Autodesk Inventor part; units mm, degrees
ref_plane "YZ Plane" through (0, 0, 0) normal (1, 0, 0) x (0, 1, 0)
ref_plane "XZ Plane" through (0, 0, 0) normal (0, 1, 0) x (-1, 0, 0)
ref_plane "XY Plane" through (0, 0, 0) normal (0, 0, 1) x (1, 0, 0)
sketch "Sketch1" plane through (0, 0, 0) normal (0, 1, 0) x (-1, 0, 0)
  circle A0 centre (0, -24) radius 19
  point P0 (0, 0)
  dimension "d1" = 38
  dimension "d3" = 24
extrude "Extrusion1" add sketch "Sketch1" along normal blind 1
sketch "Sketch3" plane through (0, 1, -24) normal (0, 1, 0) x (1, 0, 0)
  circle A0 centre (0, 0) radius 14
  circle A1 centre (0, 0) radius 19
  circle A2 centre (0, 0) radius 19
  point P0 (0, -24)
  dimension "d7" = 28
extrude "Extrusion3" add sketch "Sketch3" along normal blind 22 contours A0
sketch "Sketch5" plane through (0, 23, -24) normal (0, 1, 0) x (1, 0, 0)
  circle A0 centre (0, 0) radius 19
  point P0 (0, -24)
extrude "Extrusion5" add sketch "Sketch5" along normal blind 1
properties part number "flywheels"
Verification items for the finished model (mm, model axes). A direction names the side the tool comes from. Coordinates: 2 decimals unless noted, no trailing zeros. Loops run counter-clockwise (first coordinate to the right, second up) from the corner with the lowest first, then second, coordinate; pieces in that order, holes last. Notation, with made-up numbers: (2.5, 55) -> (13.5, 55) arc R25 ccw to (13.5, 73) -> close; hole circle Ø2 at (-30, 68.5). An arc over 180 degrees is marked (long way). Answer in a Markdown table with one row per item. Add a question column.
1. Access from +Z, -Z, +X, -X, +Y, -Y to the whole of each face (thin tool, end or side, straight path). Record for faces 1 (the face through (9, 1, -35)), 2 (the face through (0, 24, -24)).
2. Section check D-D, the plane z = -9. Enter the section's corners in (x, y).
3. Section check B-B, the plane x = 0. Enter the section's corners in (y, z).
4. Draft check along Y on faces 3 (the face through (-3.03, 11.85, -37.67)), 4 (the face through (0, 0, -24)), 5 (the face through (-10.214, 0.493, -40.021)). Enter one of: +Y half, -Y half, draft (parallel to the pull), parting line (faces both ways), or undercut.
5. Section check C-C, the plane y = 16.5. Enter the section's corners in (x, z).
6. Section check A-A, the plane z = -24. Enter the section's corners in (x, y), then the cut area to 3 significant figures.
7. Material ranges on probe 1 along Y at (x, z) = (9, -11); probe 2 along X at (y, z) = (12, -11); probe 3 along X at (y, z) = (19.5, -29), recorded low to high. Write a range as [from, to].
8. Depth check by flat-ended pin: P1, Ø1, axis at y = 8.5, z = -33.5, coming from the +X side; P2, Ø4, axis at x = 10.5, y = 5, coming from the -Z side; P3, Ø3, axis at y = 7.5, z = -21.5, coming from the -X side. Enter the tip coordinate at first touch or a pass-through.
Derived:
| question | item | result |
|---|---|---|
| 1 | face 1 | none |
| 1 | face 2 | +Z, -Z, +X, -X, +Y |
| 2 | outline | (-11.66, 0) -> (11.66, 0) -> (11.66, 1) -> (-11.66, 1) -> close; (-11.66, 23) -> (11.66, 23) -> (11.66, 24) -> (-11.66, 24) -> close |
| 3 | outline | (0, -43) -> (1, -43) -> (1, -38) -> (23, -38) -> (23, -43) -> (24, -43) -> (24, -5) -> (23, -5) -> (23, -10) -> (1, -10) -> (1, -5) -> (0, -5) -> close |
| 4 | face 3 | undercut |
| 4 | face 4 | -Y half |
| 4 | face 5 | draft |
| 5 | outline | circle Ø28 at (0, -24) |
| 6 | outline | (-19, 0) -> (19, 0) -> (19, 1) -> (14, 1) -> (14, 23) -> (19, 23) -> (19, 24) -> (-19, 24) -> (-19, 23) -> (-14, 23) -> (-14, 1) -> (-19, 1) -> close |
| 6 | area | 692 mm² |
| 7 | probe 1 | y = [0, 1], [23, 24] |
| 7 | probe 2 | x = [-5.2, 5.2] |
| 7 | probe 3 | x = [-13.08, 13.08] |
| 8 | P1 | stops at x = 10.72 |
| 8 | P2 | stops at z = -35.12 |
| 8 | P3 | stops at x = -13.96 |
